Geometry: final body of the model. Coordinates: model frame, mm. A direction names the side the tool comes from. Give positions to 0.01 mm unless a question says otherwise; leave off trailing zeros. Write each loop counter-clockwise with the first axis right and the second up, starting at its lowest first coordinate (ties: lowest second). Pieces come first, ordered by that corner, then holes. Notation, with made-up numbers: (-21, 17) -> (26, 17) arc R5 ccw to (26, 23) -> close; hole circle Ø5 at (78.25, 72.5). An arc over 180 degrees is marked (long way). Answer as a JSON object with one key per item and string values. Group by question number.
(1) Section query D-D on z = -1. Output: boundary loops of the cut face in (x, y).
(2) Material intervals for probe 1 along Y at (x, z) = (0, 9); probe 2 along Y at (x, z) = (0, 13.15); probe 3 along Z at (x, y) = (-0.25, 1.75), sorted ascending.
(3) Section query A-A on y = -6. Output: boundary loops of the cut face in (x, z).
(4) Set-up query: faces 1 (the face through (-1, -6, 0)), 2 (the face through (0, 0, 5)), 3 (the face through (0, 5.5, 0)). Return all of +Z, -Z, +X, -X, +Y, -Y with unobstructed straight access to the full face (end or side cutting, diameter ignored); none if empty.
(5) Contact query for flat-ended pins moving along their axis: pin 1 Ø8 at (x, z) = (-5.5, 1) entering from +Y; pin 2 Ø3 at (x, z) = (-4, 6) entering from -Y; pin 3 Ø4 at (x, z) = (5.5, 4) entering from +Y. Output: stop coordinate, or through.
(6) Section query C-C on z = 9. Output: boundary loops of the cut face in (x, y), plus the area to 3 significant figures.
(7) Section query B-B on x = 0. Output: boundary loops of the cut face in (y, z).
(8) Draft query along X for faces 4 (the face through (-1.8, -3.2, 5)), 5 (the face through (0, 1.55, 8)), 6 (the face through (7.5, -0.15, 0.07)). Return one class per face: +X half, -X half, draft (parallel to the pull), parting line (faces both ways), or undercut.
from build123d import *
from build123d.topology import SkipClean

# Parameters (mm, degrees)
SKETCH_1_R               = 7.5
EXTRUDE_1_DEPTH          = 5
SKETCH_6_R               = 3.5
EXTRUDE_2_DEPTH          = 10
SKETCH_7_R               = 2
CUT_EXTRUDE_1_DEPTH      = 3
CUT_EXTRUDE_2_DEPTH      = 21.03746491
CUT_EXTRUDE_2_DEPTH_BACK = 7
SKETCH_10_W              = 2
SKETCH_10_H              = 2
CUT_EXTRUDE_4_DEPTH      = 10


with BuildPart() as part:
    # Эскиз1 → Бобышка-Вытянуть1 (new, symmetric)
    with BuildSketch(Plane.XY):
        Circle(SKETCH_1_R)
    extrude(amount=EXTRUDE_1_DEPTH, both=True)

    # Эскиз6 → Бобышка-Вытянуть2 (add)
    with BuildSketch(Plane.XY.offset(5)):
        Circle(SKETCH_6_R)
    extrude(amount=EXTRUDE_2_DEPTH)

    # Эскиз7 → Вырез-Вытянуть1 (cut)
    with BuildSketch(Plane.XY.offset(15)):
        Circle(SKETCH_7_R)
    extrude(amount=-CUT_EXTRUDE_1_DEPTH, mode=Mode.SUBTRACT)

    # Эскиз8 → Вырез-Вытянуть2 (cut, two sides: drawn at the far end of the back side and taken through both)
    with SkipClean():  # the faces are left unmerged after this step: merging them gives an invalid solid
        with BuildSketch(Plane.XY.offset(12).offset(-CUT_EXTRUDE_2_DEPTH_BACK)):
            with BuildLine():
                Line((1.263922466, 1.55), (-1.263922466, 1.55))
                ThreePointArc((-1.263922466, 1.55), (-0.85794961, -1.806632908), (2, 0))
                ThreePointArc((2, 0), (1.806632908, 0.85794961), (1.263922466, 1.55))
            make_face()
        extrude(amount=CUT_EXTRUDE_2_DEPTH + CUT_EXTRUDE_2_DEPTH_BACK, mode=Mode.SUBTRACT)

    # Эскиз10 → Вырез-Вытянуть4 (cut)
    with SkipClean():  # the faces are left unmerged after this step: merging them gives an invalid solid
        with BuildSketch(Plane.XY.offset(5)):
            with Locations((0, 6.5)):
                Rectangle(SKETCH_10_W, SKETCH_10_H)
            with Locations((0, -6.5)):
                Rectangle(SKETCH_10_W, SKETCH_10_H)
        extrude(amount=-CUT_EXTRUDE_4_DEPTH, mode=Mode.SUBTRACT)


solid = part.part
Answer list:
{
 "1": {"outline": "(-1, -7.43) -> (-1, -5.5) -> (1, -5.5) -> (1, -7.43) arc R7.5 ccw to (1, 7.43) -> (1, 5.5) -> (-1, 5.5) -> (-1, 7.43) arc R7.5 ccw to start"},
 "2": {"probe 1": "-3.5 to -2, 1.55 to 3.5", "probe 2": "-3.5 to -2, 2 to 3.5", "probe 3": "-5 to 12"},
 "3": {"outline": "(-4.5, -5) -> (-1, -5) -> (-1, 5) -> (-4.5, 5) -> close; (1, -5) -> (4.5, -5) -> (4.5, 5) -> (1, 5) -> close"},
 "4": {"face 1": "+Z, -Z, -Y", "face 2": "+Z", "face 3": "+Z, -Z, +Y"},
 "5": {"pin 1": "y = 7.35", "pin 2": "y = -6.92", "pin 3": "y = 6.63"},
 "6": {"outline": "circle Ø7 at (0, 0); hole (-1.26, 1.55) arc R2 ccw (long way) to (1.26, 1.55) -> close", "area": "26.7 mm2"},
 "7": {"outline": "(-5.5, -5) -> (5.5, -5) -> (5.5, 5) -> (3.5, 5) -> (3.5, 15) -> (2, 15) -> (2, 12) -> (1.55, 12) -> (1.55, 5) -> (-2, 5) -> (-2, 15) -> (-3.5, 15) -> (-3.5, 5) -> (-5.5, 5) -> close"},
 "8": {"face 4": "draft", "face 5": "undercut", "face 6": "+X half"}
}
